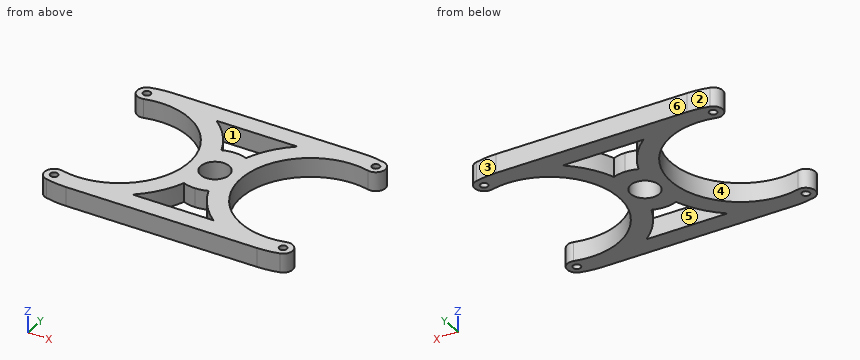
```python
from build123d import *

# Parameters (mm, degrees)
F0_R     = 2
F1_DEPTH = 10


with BuildPart() as f1:
    # F0 (on Top) → F1 (new body)
    with BuildSketch(Plane.XY):
        with BuildLine():
            ThreePointArc((58.795181, -35.424494), (13.5, 0), (58.795181, 35.424494))
            ThreePointArc((58.795181, 35.424494), (64.85267, 39.072345), (61.204819, 45.129835))
            ThreePointArc((61.204819, 45.129835), (55.644141, 46.156188), (50, 46.5))
            Line((50, 46.5), (0, 46.5))
            Line((0, 46.5), (-50, 46.5))
            ThreePointArc((-50, 46.5), (-55.644141, 46.156188), (-61.204819, 45.129835))
            ThreePointArc((-61.204819, 45.129835), (-64.85267, 39.072345), (-58.795181, 35.424494))
            ThreePointArc((-58.795181, 35.424494), (-13.5, 0), (-58.795181, -35.424494))
            ThreePointArc((-58.795181, -35.424494), (-64.85267, -39.072345), (-61.204819, -45.129835))
            ThreePointArc((-61.204819, -45.129835), (-55.644141, -46.156188), (-50, -46.5))
            Line((-50, -46.5), (0, -46.5))
            Line((0, -46.5), (50, -46.5))
            ThreePointArc((50, -46.5), (55.644141, -46.156188), (61.204819, -45.129835))
            ThreePointArc((61.204819, -45.129835), (64.85267, -39.072345), (58.795181, -35.424494))
        make_face()
        with Locations((-60, -40.277165)):
            Circle(F0_R, mode=Mode.SUBTRACT)
        with BuildLine():
            ThreePointArc((0, -17.5), (3.278022, -17.190247), (6.44, -16.271951))
            ThreePointArc((6.44, -16.271951), (12.428234, -27.397306), (21.190279, -36.5))
            Line((21.190279, -36.5), (0, -36.5))
            Line((0, -36.5), (-21.190279, -36.5))
            ThreePointArc((-21.190279, -36.5), (-12.428234, -27.397306), (-6.44, -16.271951))
            ThreePointArc((-6.44, -16.271951), (-3.278022, -17.190247), (0, -17.5))
        make_face(mode=Mode.SUBTRACT)
        with Locations((60, -40.277165)):
            Circle(F0_R, mode=Mode.SUBTRACT)
        with Locations((-60, 40.277165)):
            Circle(F0_R, mode=Mode.SUBTRACT)
        with BuildLine():
            ThreePointArc((0, 7.5), (7.5, 0), (0, -7.5))
            ThreePointArc((0, -7.5), (-7.5, 0), (0, 7.5))
        make_face(mode=Mode.SUBTRACT)
        with BuildLine():
            ThreePointArc((21.190279, 36.5), (12.428234, 27.397306), (6.44, 16.271951))
            ThreePointArc((6.44, 16.271951), (3.278022, 17.190247), (0, 17.5))
            ThreePointArc((0, 17.5), (-3.278022, 17.190247), (-6.44, 16.271951))
            ThreePointArc((-6.44, 16.271951), (-12.428234, 27.397306), (-21.190279, 36.5))
            Line((-21.190279, 36.5), (0, 36.5))
            Line((0, 36.5), (21.190279, 36.5))
        make_face(mode=Mode.SUBTRACT)
        with Locations((60, 40.277165)):
            Circle(F0_R, mode=Mode.SUBTRACT)
    extrude(amount=F1_DEPTH)


solid = f1.part
```
CAD build for the part. Positions are in the model's coordinates, mm. Face numbers are marked on the shaded views. A direction names the side the tool comes from. Round coordinates to 2 decimals unless told otherwise and drop trailing zeros. Write each loop counter-clockwise with the first axis right and the second up, starting at its lowest first coordinate (ties: lowest second). Pieces come first, ordered by that corner, then holes. Notation, with made-up numbers: (3.25, 26) -> (32.25, 26) arc R17 ccw to (32.25, 51) -> close; hole circle Ø7 at (7.5, -11.5). An arc over 180 degrees is marked (long way). Answer in a Markdown table with one row per item. Add a question column.
Item 1: Mould opens along X. For the marked faces 1, 2, 3 and 4 say: pulls with the +X half, pulls with the -X half, needs draft (parallel to the pull), parting line crosses it, or undercut.
Item 2: Which spindle directions (+Z, -Z, +X, -X, +Y, -Y) get a long thin tool onto all of the face, cutting with end or side? Do the marked faces 5 and 6. Say none if no direction does.
Item 3: Saw through at C-C, the plane z = 5.5. Write the cut outline in (x, y).
Item 4: Drill centre lines: line 1 (Y direction, x = -0.5, z = 6.25); line 2 (X direction, y = -40.5, z = 8.25); line 3 (Y direction, x = 50, z = 7). Where is each one in solid material? Low to high. Write a range as from..to.
Item 5: Saw through at A-A, the plane y = 0. Write the cut outline in (x, z).
Item 6: Drop flat-ended pins along their axis: pin 1 Ø1.5 at (y, z) = (-2.5, 5.5) entering from -X (3 decimals); pin 2 Ø3 at (y, z) = (23, 3.5) entering from -X. Give the stop position or say it passes through.
Item 7: Saw through at B-B, the plane x = -41. Write the cut outline in (y, z), then the cut area to 3 significant figures.
Findings below:
| question | item | result |
|---|---|---|
| 1 | face 1 | undercut |
| 1 | face 2 | pulls with the -X half |
| 1 | face 3 | pulls with the +X half |
| 1 | face 4 | undercut |
| 2 | face 5 | +Z, -Z |
| 2 | face 6 | +Z, -Z, +X, -X, +Y |
| 3 | outline | (-61.2, -45.13) arc R46.5 ccw to (-50, -46.5) -> (50, -46.5) arc R46.5 ccw to (61.2, -45.13) arc R5 ccw to (58.8, -35.42) arc R36.5 cw (long way) to (58.8, 35.42) arc R5 ccw to (61.2, 45.13) arc R46.5 ccw to (50, 46.5) -> (-50, 46.5) arc R46.5 ccw to (-61.2, 45.13) arc R5 ccw to (-58.8, 35.42) arc R36.5 cw (long way) to (-58.8, -35.42) arc R5 ccw to start; hole circle Ø4 at (-60, -40.28); hole circle Ø4 at (-60, 40.28); hole (-21.19, -36.5) -> (21.19, -36.5) arc R46.5 cw to (6.44, -16.27) arc R17.5 cw to (0, -17.5) arc R17.5 cw to (-6.44, -16.27) arc R46.5 cw to start; hole (-21.19, 36.5) arc R46.5 cw to (-6.44, 16.27) arc R17.5 cw to (0, 17.5) arc R17.5 cw to (6.44, 16.27) arc R46.5 cw to (21.19, 36.5) -> close; hole circle Ø15 at (0, 0); hole circle Ø4 at (60, -40.28); hole circle Ø4 at (60, 40.28) |
| 4 | line 1 | y = -46.5..-36.5, -17.49..-7.48, 7.48..17.49, 36.5..46.5 |
| 4 | line 2 | x = -65..-61.99, -58.01..58.01, 61.99..65 |
| 4 | line 3 | y = -46.5..-36.5, 36.5..46.5 |
| 5 | outline | (-13.5, 0) -> (-7.5, 0) -> (-7.5, 10) -> (-13.5, 10) -> close; (7.5, 0) -> (13.5, 0) -> (13.5, 10) -> (7.5, 10) -> close |
| 6 | pin 1 | stops at x = -13.645 |
| 6 | pin 2 | stops at x = -22.94 |
| 7 | outline | (-46.5, 0) -> (-35.37, 0) -> (-35.37, 10) -> (-46.5, 10) -> close; (35.37, 0) -> (46.5, 0) -> (46.5, 10) -> (35.37, 10) -> close |
| 7 | area | 223 mm^2 |
